Autodesk Inventor part; units mm, degrees
ref_plane "YZ Plane" through (0, 0, 0) normal (1, 0, 0) x (0, 1, 0)
ref_plane "XZ Plane" through (0, 0, 0) normal (0, 1, 0) x (-1, 0, 0)
ref_plane "XY Plane" through (0, 0, 0) normal (0, 0, 1) x (1, 0, 0)
sketch "Sketch3" plane through (0, 0, 0) normal (0, 1, 0) x (-1, 0, 0)
  line L0 (0.75, -50) -> (-0.75, -50)
  line L1 (-0.75, -50) -> (-0.75, 50)
  line L2 (-0.75, 50) -> (0.75, 50)
  line L3 (0.75, 50) -> (0.75, -50)
  line L4 (0.75, -50) -> (-0.75, 50) construction
  line L5 (-0.75, -50) -> (0.75, 50) construction
  line L6 (0.75, -50) -> (0.75, -30)
  line L7 (0.75, -30) -> (5.75, -30)
  line L8 (5.75, -30) -> (5.75, -50)
  line L9 (5.75, -50) -> (0.75, -50)
  line L10 (0.75, -30) -> (6.2137, -30) construction
  line L11 (0.75, -50) -> (5.75, -47.1132)
  line L12 (0.75, -50) -> (6.5235, -50) construction
  line L13 (0.75, -30) -> (5.75, -32.8868)
  line L14 (0.75, -30) -> (5.6279, -30) construction
  line L15 (0.75, -28) -> (5.75, -25.1132)
  line L16 (5.75, -8) -> (5.75, -28)
  line L17 (0.75, -8) -> (5.75, -10.8868)
  line L18 (0.75, -6) -> (5.75, -3.1132)
  line L19 (5.75, 14) -> (5.75, -6)
  line L20 (0.75, 14) -> (5.75, 11.1132)
  line L21 (0.75, 16) -> (5.75, 18.8868)
  line L22 (5.75, 36) -> (5.75, 16)
  line L23 (0.75, 36) -> (5.75, 33.1132)
  line L24 (-0.75, 50) -> (0.75, 50)
  line L25 (0.75, 50) -> (0.75, 80)
  line L26 (0.75, 80) -> (-0.75, 80)
  line L27 (-0.75, 80) -> (-0.75, 50)
  line L28 (-1.5102, -55) -> (-1.5102, 40) construction
  line L29 (-0.5, 40) -> (-0.6183, 40) construction
  point P0 (0, 0)
  point P1 (0.75, 14)
  point P2 (0.75, -8)
  point P3 (0.75, -28)
  point P4 (-1.5102, -45.1132)
  point P5 (-1.5102, -34.8868)
  point P6 (-1.5102, -12.8868)
  point P7 (-1.5102, -23.1132)
  point P8 (-1.5102, 9.1132)
  point P9 (-1.5102, -1.1132)
  point P10 (-1.5102, 31.1132)
  point P11 (-1.5102, 20.8868)
  point P12 (5.75, 26)
  point P13 (5.75, 4)
  dimension "d17" = 1.5
  dimension "d18" = 100
  dimension "d19" = 20
  dimension "d20" = 5
  dimension "d22" = 30
  dimension "d23" = 30
  dimension "d26" = 22
  dimension "d35" = 1.5
  dimension "d36" = 30
  dimension "d61" = 95
  dimension "d62" = 2
  dimension "d63" = 2
  dimension "d66" = 22
  dimension "d74" = 22
  dimension "d75" = 130
extrude "Extrusion1" add sketch "Sketch3" along normal mid plane 12 contours L0 L1 L2 L3 | L27 L26 L25 L2
extrude "Extrusion2" add sketch "Sketch3" along normal mid plane 6 contours L3 L13 L8 L11 | L3 L17 L16 L15 | L23 L22 L21 L3 | L3 L20 L19 L18
sketch "Sketch4" plane through (-0.75, -6, 80) normal (-1, 0, 0) x (0, 0, 1)
  circle A0 centre (-32, 6) radius 2
  line L0 (-44, 9) -> (-44, 3)
  line L1 (-44, 6) -> (0, 6) construction
  line L2 (0, 12) -> (0, 0) construction
  circle A1 centre (-25, 6) radius 2
  circle A2 centre (-18, 6) radius 2
  circle A3 centre (-11, 6) radius 2
  circle A4 centre (-4, 6) radius 2
  point P0 (-80, 6)
  dimension "d37" = 4
  dimension "d38" = 12
  dimension "d41" = 7
extrude "Extrusion3" cut sketch "Sketch4" against normal blind 6
sketch "Sketch5" plane through (-0.75, 6, 80) normal (0, 0, 1) x (1, 0, 0)
  line L0 (-5, -9) -> (-5, -3) construction
  line L1 (0, -9) -> (0, -3) construction
  line L2 (-5, -9) -> (0, -9) construction
  line L3 (0, -9) -> (0, -3) construction
  line L4 (0, -3) -> (-5, -3) construction
  line L5 (-5, -3) -> (-5, -9) construction
  line L6 (0, -9) -> (-5, -3) construction
  line L7 (-5, -9) -> (0, -3) construction
  line L8 (-2.5, -6) -> (-3.6, -6) construction
  line L9 (-3.6, -6) -> (-3.6, -7) construction
  circle A0 centre (-3.6, -7) radius 0.5
  circle A1 centre (-3.6, -5) radius 0.5
  point P0 (0.75, -6)
  dimension "d48" = 6
  dimension "d49" = 1.1
  dimension "d58" = 1
  dimension "d59" = 1
extrude "Extrusion4" cut sketch "Sketch5" against normal blind 150
fillet "Fillet1" radius 1 4 edges at (0, 6, 80) (0, -6, 80) (0, -6, -50) (0, 6, -50)
sketch "Sketch6" plane through (-0.75, -3, -50) normal (0, 0, -1) x (-1, 0, 0)
  line L0 (-1.5, 1) -> (-1.5, 5)
  circle A0 centre (-1.5, 3) radius 1
  point P0 (-0.75, 3)
  point P1 (-2, 4)
  point P2 (-2, 2)
  dimension "d71" = 2
properties part number "actuator_bone_joint"
Geometry check sheet. Reference: the model listing, model coordinates, mm. A direction names the side the tool comes from. Round coordinates to 2 decimals unless told otherwise and drop trailing zeros. Order: outer loops, then holes, each group sorted by start corner. A loop starts at its lowest first (then second) coordinate and runs counter-clockwise, first axis right, second up. Notation, with made-up numbers: (8.5, 68.5) - (66.5, 68.5) arc R12 cw to (66.5, 84.5) - close; hole circle Ø2 at (48.25, 80). An arc over 180 degrees is marked (long way). Use a Markdown table: item, result. Add a question column.
1) Set-up check for faces 5 (the flat face through (-3, 3, -18)), 6 (the flat face through (-3, -3, 4)), 7 (the flat face through (-3.215, -0.042, -31.423)): record each of +Z, -Z, +X, -X, +Y, -Y from which the full face is reachable in a straight line by a thin tool's end or side.
2) Section check C-C (x = -2). Record the cut outline in (y, z), then the cut area to 3 significant figures.
3) Section check A-A (z = 62). Record the cut outline in (x, y).
4) Gauge pin test, flat ends, axial feed: P1, Ø2, axis at x = -5, y = 4.5, coming from the +Z side; P2, Ø5, axis at y = 0, z = 48, coming from the -X side; P3, Ø1.5, axis at x = -4.5, z = -19.5, coming from the +Y side; P4, Ø1.5, axis at x = -3, z = -37, coming from the -Y side. Record the tip position at first contact, or that the pin passes through.
5) Mould release check, pull along Z, two halves, no side actions. Record for faces 1 (the flat face through (-3.215, -0.042, -48.577)), 2 (the flat face through (-3.215, -0.042, 34.577)), 3 (the flat face through (-5.75, 0, 26)), 4 (the cylindrical face through (0, 0, 46)): released by +Z, released by -Z, zero draft, split by the parting line, or undercut.
6) Section check D-D (z = 42.5). Record the cut outline in (x, y), then the cut area to 3 significant figures.
7) Section check B-B (z = 5.5). Record the cut outline in (x, y).
8) Thickness scan on line 1 along Y through (x, z) = (-4.35, -22.25); line 2 along Z through (x, y) = (-1.5, 0.75); line 3 along Z through (x, y) = (-2, 2.75). Record the ranges inside material, lowest first.
Established:
| question | item | result |
|---|---|---|
| 1 | face 5 | +Z, -Z, -X, +Y |
| 1 | face 6 | +Z, -Z, -X, -Y |
| 1 | face 7 | -X, +Y, -Y |
| 2 | outline | (-3, -49.28) - (3, -49.28) - (3, -30.72) - (-3, -30.72) - close; (-3, -27.28) - (3, -27.28) - (3, -8.72) - (-3, -8.72) - close; (-3, -5.28) - (3, -5.28) - (3, 13.28) - (-3, 13.28) - close; (-3, 16.72) - (3, 16.72) - (3, 35.28) - (-3, 35.28) - close |
| 2 | area | 445 mm2 |
| 3 | outline | (-0.75, -6) - (0.75, -6) - (0.75, -2) - (-0.75, -2) - close; (-0.75, 2) - (0.75, 2) - (0.75, 6) - (-0.75, 6) - close |
| 4 | P1 | through |
| 4 | P2 | x = -0.75 |
| 4 | P3 | y = 3 |
| 4 | P4 | y = -3 |
| 5 | face 1 | released by -Z |
| 5 | face 2 | released by +Z |
| 5 | face 3 | zero draft |
| 5 | face 4 | undercut |
| 6 | outline | (-0.75, -6) - (0.75, -6) - (0.75, 6) - (-0.75, 6) - close |
| 6 | area | 18.0 mm2 |
| 7 | outline | (-5.75, -3) - (-0.75, -3) - (-0.75, -6) - (0.75, -6) - (0.75, 6) - (-0.75, 6) - (-0.75, 3) - (-5.75, 3) - close; hole circle Ø1 at (-4.35, -1); hole circle Ø1 at (-4.35, 1) |
| 8 | line 1 | -3 to -1.5, -0.5 to 0.5, 1.5 to 3 |
| 8 | line 2 | -49.57 to -30.43, -27.57 to -8.43, -5.57 to 13.57, 16.43 to 35.57 |
| 8 | line 3 | -49.28 to -30.72, -27.28 to -8.72, -5.28 to 13.28, 16.72 to 35.28 |
